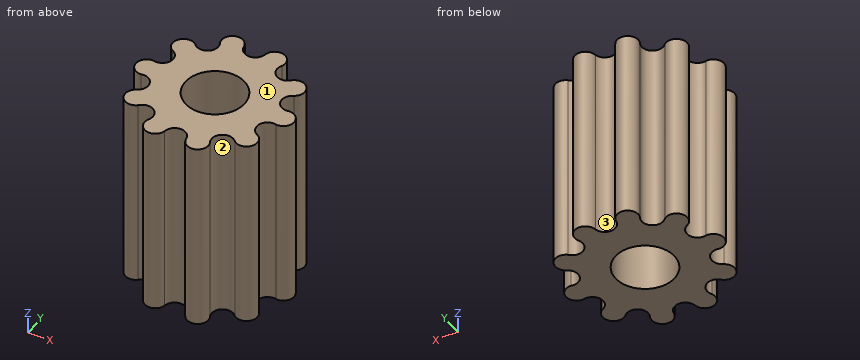
from build123d import *

# Parameters (mm, degrees)
EXTRUDE001_DEPTH = 2
SKETCH_R         = 2.6
EXTRUDE_DEPTH    = 8.5


with BuildPart() as nut_pocket:
    # Sketch001 → Extrude001 (new body, symmetric)
    with BuildSketch(Plane.XY):
        Polygon((-4.835, 0), (-2.4, -4.2), (2.4, -4.2), (4.835, 0), (2.4, 4.2), (-2.4, 4.2), align=None)
    extrude(amount=EXTRUDE001_DEPTH, both=True)


with BuildPart() as cut:
    # Sketch → Extrude (new body, symmetric)
    with BuildSketch(Plane.XY):
        with BuildLine():
            ThreePointArc((-0.938607, 5.92613), (-0.07387, 5.061393), (0.915495, 5.780209))
            ThreePointArc((2.723943, 5.346039), (2.073893, 6.621834), (0.915495, 5.780209))
            ThreePointArc((2.723943, 5.346039), (2.973306, 4.092405), (4.242641, 4.242641))
            ThreePointArc((5.346039, 2.723943), (5.615799, 4.080117), (4.242641, 4.242641))
            ThreePointArc((5.346039, 2.723943), (4.810911, 1.56316), (5.92613, 0.938607))
            ThreePointArc((5.92613, -0.938607), (6.941509, 0), (5.92613, 0.938607))
            ThreePointArc((5.92613, -0.938607), (4.810911, -1.56316), (5.346039, -2.723943))
            ThreePointArc((4.242641, -4.242641), (5.615799, -4.080117), (5.346039, -2.723943))
            ThreePointArc((4.242641, -4.242641), (2.973306, -4.092405), (2.723943, -5.346039))
            ThreePointArc((0.938607, -5.92613), (2.145044, -6.601768), (2.723943, -5.346039))
            ThreePointArc((0.938607, -5.92613), (0, -5.058491), (-0.938607, -5.92613))
            ThreePointArc((-2.723943, -5.346039), (-2.145044, -6.601768), (-0.938607, -5.92613))
            ThreePointArc((-2.723943, -5.346039), (-2.973306, -4.092405), (-4.242641, -4.242641))
            ThreePointArc((-5.346039, -2.723943), (-5.615799, -4.080117), (-4.242641, -4.242641))
            ThreePointArc((-5.346039, -2.723943), (-4.810911, -1.56316), (-5.92613, -0.938607))
            ThreePointArc((-5.92613, 0.938607), (-6.941509, 0), (-5.92613, -0.938607))
            ThreePointArc((-5.92613, 0.938607), (-4.810911, 1.56316), (-5.346039, 2.723943))
            ThreePointArc((-4.242641, 4.242641), (-5.615799, 4.080117), (-5.346039, 2.723943))
            ThreePointArc((-4.242641, 4.242641), (-2.973306, 4.092405), (-2.723943, 5.346039))
            ThreePointArc((-0.938607, 5.92613), (-2.145044, 6.601768), (-2.723943, 5.346039))
        make_face()
        Circle(SKETCH_R, mode=Mode.SUBTRACT)
    extrude(amount=EXTRUDE_DEPTH, both=True)

    # Cut: cut Nut Pocket
    add(nut_pocket.part, mode=Mode.SUBTRACT)


solid = cut.part
Verification items for the finished model (mm, model axes). Face numbers are marked on the shaded views. Round coordinates to 2 decimals unless told otherwise and drop trailing zeros. Write each loop counter-clockwise with the first axis right and the second up, starting at its lowest first coordinate (ties: lowest second). Pieces come first, ordered by that corner, then holes.
(1) Section check C-C (x = -4.5). Enter the section's corners in (y, z), plus the area to 3 significant figures.
Returned:
outline: (-4.4, -8.5) - (4.4, -8.5) - (4.4, 8.5) - (-4.4, 8.5) - close; hole (-0.58, -2) - (0.58, -2) - (0.58, 2) - (-0.58, 2) - close
area: 145 mm2
(2) Section check A-A (x = 0). Enter the section's corners in (y, z).
Returned:
outline: (-5.06, -8.5) - (-2.6, -8.5) - (-2.6, -2) - (-4.2, -2) - (-4.2, 2) - (-2.6, 2) - (-2.6, 8.5) - (-5.06, 8.5) - close; (2.6, -8.5) - (5.06, -8.5) - (5.06, 8.5) - (2.6, 8.5) - (2.6, 2) - (4.2, 2) - (4.2, -2) - (2.6, -2) - close
(3) Depth check by flat-ended pin: pin 1 Ø3 at (x, z) = (-5, -5) entering from -Y; pin 2 Ø1.2 at (x, z) = (-0.5, -0.5) entering from -Y; pin 3 Ø1 at (y, z) = (4, 2) entering from -X; pin 4 Ø4 at (x, y) = (0, 0) entering from -Z. Enter the tip coordinate at first touch or a pass-through.
Returned:
pin 1: stops at y = -4.47
pin 2: stops at y = -6.27
pin 3: stops at x = -5.8
pin 4: passes through
(4) Mould release check, pull along Y, two halves, no side actions. Record for the marked faces 1, 2 and 3: pulls with the +Y half, pulls with the -Y half, needs draft (parallel to the pull), parting line crosses it, or undercut.
Returned:
face 1: needs draft
face 2: undercut
face 3: pulls with the +Y half
(5) Material ranges on line 1 (Z direction, x = -1.75, y = 3.25); line 2 (Y direction, x = 6, z = -1); line 3 (Y direction, x = 0, z = -4), recorded low to high.
Returned:
line 1: z = -8.5 to -2, 2 to 8.5
line 2: y = -0.94 to 0.94
line 3: y = -5.06 to -2.6, 2.6 to 5.06
(6) Section check B-B (y = -2). Enter the section's corners in (x, z), plus the area to 3 significant figures.
Returned:
outline: (-4.78, -8.5) - (-1.66, -8.5) - (-1.66, -2) - (-3.68, -2) - (-3.68, 2) - (-1.66, 2) - (-1.66, 8.5) - (-4.78, 8.5) - close; (1.66, -8.5) - (4.78, -8.5) - (4.78, 8.5) - (1.66, 8.5) - (1.66, 2) - (3.68, 2) - (3.68, -2) - (1.66, -2) - close
area: 89.8 mm2
